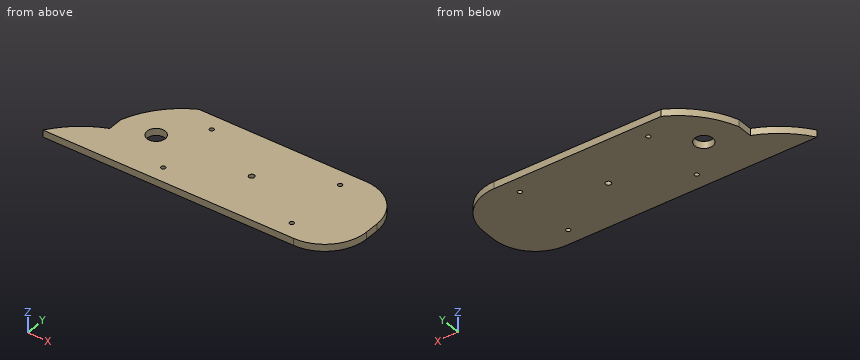
```python
from build123d import *

# Parameters (mm, degrees)
BOSS_EXTRUDE1_DEPTH = 12.7
SKETCH4_R           = 5.08
SKETCH4_R_2         = 3.937
SKETCH4_R_3         = 16.51
CUT_EXTRUDE2_DEPTH  = 563.396381567


with BuildPart() as part:
    # Sketch2 → Boss-Extrude1 (new body)
    with BuildSketch(Plane.XY):
        with BuildLine():
            Line((0, 0), (457.2, 0))
            ThreePointArc((457.2, 0), (511.081536726, 22.318463274), (533.4, 76.2))
            Line((533.4, 76.2), (533.4, 101.6))
            ThreePointArc((533.4, 101.6), (511.081536726, 155.481536726), (457.2, 177.8))
            Line((457.2, 177.8), (152.4, 177.8))
            ThreePointArc((152.4, 177.8), (105.657968509, 140.757455564), (76.2, 88.9))
            Line((76.2, 88.9), (76.2, 61.401251199))
            ThreePointArc((76.2, 61.401251199), (33.506060073, 36.401783403), (0, 0))
        make_face()
    extrude(amount=BOSS_EXTRUDE1_DEPTH)

    # Sketch4 → Cut-Extrude2 (cut, through all)
    with BuildSketch(Plane.XY.offset(12.7)):
        with Locations((314.706, 88.9)):
            Circle(SKETCH4_R)
        with Locations((431.8, 148.4376)):
            Circle(SKETCH4_R_2)
        with Locations((140.468339853, 88.9)):
            Circle(SKETCH4_R_3)
        with Locations(Location((197.612, 148.4376, 0), (0, 0, 180))):
            Circle(SKETCH4_R_2)
        with Locations((197.612, 29.3624)):
            Circle(SKETCH4_R_2)
        with Locations(Location((431.8, 29.3624, 0), (0, 0, 180))):
            Circle(SKETCH4_R_2)
    extrude(amount=-CUT_EXTRUDE2_DEPTH, mode=Mode.SUBTRACT)


solid = part.part
```
Model file for the job. Use its own axes, mm. Round coordinates to 2 decimals unless told otherwise and drop trailing zeros. Write each loop counter-clockwise with the first axis right and the second up, starting at its lowest first coordinate (ties: lowest second). Pieces come first, ordered by that corner, then holes. Notation, with made-up numbers: (66, -18.5) - (77, -18.5) arc R37 cw to (77, 17.5) - close; hole circle Ø10 at (8.5, -10). An arc over 180 degrees is marked (long way). One line per item, written item: value.
(1) Cut at A-A, the plane x = 131. Give the cut face in (y, z), plus the area to 3 significant figures.
Values follow:
outline: (0, 0) - (75.37, 0) - (75.37, 12.7) - (0, 12.7) - close; (102.43, 0) - (164.41, 0) - (164.41, 12.7) - (102.43, 12.7) - close
area: 1,740 mm²
(2) Cut at D-D, the plane x = 55. Give the cut face in (y, z).
Values follow:
outline: (0, 0) - (51.12, 0) - (51.12, 12.7) - (0, 12.7) - close
(3) Wall check: probe 1 along X at (y, z) = (30, 7); probe 2 along Y at (x, z) = (431, 3); probe 3 along Y at (x, z) = (131, 11.25). Give the ranges that are in metal, low to high.
Values follow:
probe 1: x = 26.02 to 193.73, 201.5 to 427.91, 435.69 to 517.8
probe 2: y = 0 to 25.51, 33.22 to 144.58, 152.29 to 177.8
probe 3: y = 0 to 75.37, 102.43 to 164.41
(4) Cut at C-C, the plane y = 17. Give the cut face in (x, z), plus the area to 3 significant figures.
Values follow:
outline: (13.19, 0) - (505.18, 0) - (505.18, 12.7) - (13.19, 12.7) - close
area: 6,250 mm²
(5) Cut at B-B, the plane z = 10.5. Give the cut face in (x, y) (3 decimals).
Values follow:
outline: (0, 0) - (457.2, 0) arc R76.2 ccw to (533.4, 76.2) - (533.4, 101.6) arc R76.2 ccw to (457.2, 177.8) - (152.4, 177.8) arc R156.251 ccw to (76.2, 88.9) - (76.2, 61.401) arc R167.157 ccw to start; hole circle Ø33.02 at (140.468, 88.9); hole circle Ø7.874 at (197.612, 29.362); hole circle Ø7.874 at (197.612, 148.438); hole circle Ø10.16 at (314.706, 88.9); hole circle Ø7.874 at (431.8, 29.362); hole circle Ø7.874 at (431.8, 148.438)
(6) Drop flat-ended pins along their axis: P1, Ø6.5, axis at y = 79.5, z = 9, coming from the -X side; P2, Ø3, axis at y = 28, z = 5, coming from the +X side; P3, Ø6, axis at x = 95.5, z = 9, coming from the +Y side. Give the stop position or say it passes through.
Values follow:
P1: stops at x = 76.2
P2: stops at x = 517.41
P3: stops at y = 131.76
